from build123d import *

# Parameters (mm, degrees)
SKETCH_1_R          = 2
EXTRUDE_1_DEPTH     = 10
SKETCH_2_R          = 4
EXTRUDE_2_DEPTH     = 2.5
FILLET_1_R          = 1
CHAMFER_1_SIZE      = 0.5
SKETCH_3_W          = 4
SKETCH_3_H          = 1
SKETCH_3_W_2        = 1
SKETCH_3_H_2        = 4
CUT_EXTRUDE_1_DEPTH = 1
CHAMFER_2_SIZE      = 1


with BuildPart() as part:
    # 草图1 → 凸台-拉伸1 (new body)
    with BuildSketch(Plane(origin=(0, 0, 0), x_dir=(1, 0, 0), z_dir=(0, 1, 0))):
        with Locations(Location((0, 0, 0), (0, 0, 270))):
            Circle(SKETCH_1_R)
    extrude(amount=EXTRUDE_1_DEPTH)

    # 草图2 → 凸台-拉伸2 (add)
    with BuildSketch(Plane(origin=(0, 10, 0), x_dir=(1, 0, 0), z_dir=(0, 1, 0))):
        with Locations(Location((0, 0, 0), (0, 0, 270))):
            Circle(SKETCH_2_R)
    extrude(amount=EXTRUDE_2_DEPTH)

    # 圆角1
    fillet_1_edges = [part.edges().sort_by_distance(p)[0] for p in [
        (0, 12.5, -4),
    ]]
    fillet(fillet_1_edges, radius=FILLET_1_R)

    # 倒角1
    chamfer_1_edges = [part.edges().sort_by_distance(p)[0] for p in [
        (0, 0, -2),
    ]]
    chamfer(chamfer_1_edges, length=CHAMFER_1_SIZE)

    # 草图3 → 切除-拉伸-薄壁1 (cut)
    with BuildSketch(Plane(origin=(0, 12.5, 0), x_dir=(1, 0, 0), z_dir=(0, 1, 0))):
        Rectangle(SKETCH_3_W, SKETCH_3_H)
        Rectangle(SKETCH_3_W_2, SKETCH_3_H_2)
    extrude(amount=-CUT_EXTRUDE_1_DEPTH, mode=Mode.SUBTRACT)

    # 倒角2
    chamfer_2_edges = [part.edges().sort_by_distance(p)[0] for p in [
        (0, 11.5, 2),
        (2, 11.5, 0),
        (0, 11.5, -2),
        (-2, 11.5, 0),
    ]]
    chamfer(chamfer_2_edges, length=CHAMFER_2_SIZE - 0.0001)  # a hair under: the kernel refuses the full size


solid = part.part
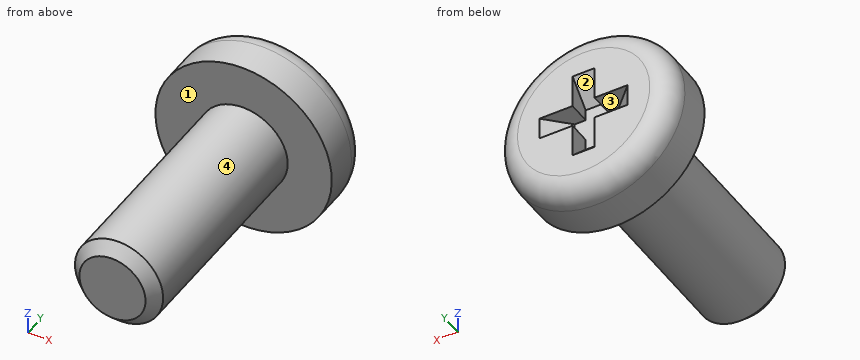
Verification items for the finished model (mm, model axes). Face numbers are marked on the shaded views. Give positions to 0.01 mm unless a question says otherwise; leave off trailing zeros. Write each loop counter-clockwise with the first axis right and the second up, starting at its lowest first coordinate (ties: lowest second). Pieces come first, ordered by that corner, then holes. Notation, with made-up numbers: M 13,78 L 34,78 A8 ccw 34,90 Z; hole C 2,-0.5 d4. An arc over 180 degrees is marked long. Use CSV: the item, a comma, the result in double quotes.
1) Release check for a two-part mould opening along X. For the marked faces 1, 2, 3 and 4 record: released by +X, released by -X, zero draft, split by the parting line, or undercut.
Final values:
face 1,"zero draft"
face 2,"undercut"
face 3,"undercut"
face 4,"split by the parting line"
2) Material ranges on line 1 along Y through (x, z) = (-2.25, 2); line 2 along X through (y, z) = (12, 0); line 3 along Z through (x, y) = (0.5, 8.25), recorded low to high.
Final values:
line 1,"10 to 12.5"
line 2,"-3.87 to -1.5, 1.5 to 3.87"
line 3,"-1.94 to 1.94"
3) Cross-section at C-C (y = 6.25). Enter the section's corners in (x, z).
Final values:
outline,"C 0,0 d4"
4) Go/stop test with flat-tipped pins: pin 1 Ø4 at (x, y) = (-1, 10) entering from -Z; pin 2 Ø0.8 at (y, z) = (12, -1.5) entering from -X; pin 3 Ø2 at (y, z) = (8, 2.5) entering from -X; pin 4 Ø0.8 at (x, y) = (1.5, 12) entering from -Z. Record where each tip stops, or that it passes through.
Final values:
pin 1,"z = -4"
pin 2,"x = -3.79"
pin 3,"x = -1.32"
pin 4,"z = -3.79"
